from build123d import *

# Parameters (mm, degrees)
SKETCH_1_W                  = 600
SKETCH_1_H                  = 600
EXTRUDE_1_DEPTH             = 780
FILLET_1_R                  = 30
SHELL_1_T                   = 1.2
SKETCH_13_W                 = 348.8
SKETCH_13_H                 = 520
CUT_EXTRUDE_6_DEPTH         = 10
SKETCH_15_W                 = 351.2
SKETCH_15_H                 = 522.4
SKETCH_15_W_2               = 348.8
SKETCH_15_H_2               = 520
EXTRUDE_7_DEPTH             = 15
SKETCH_16_W                 = 351.2
SKETCH_16_H                 = 522.4
SKETCH_16_W_2               = 331.2
SKETCH_16_H_2               = 502.4
EXTRUDE_8_DEPTH             = 1.2
SKETCH_17_W                 = 680
SKETCH_17_H                 = 520
CUT_EXTRUDE_7_DEPTH         = 1.2
SKETCH_19_W                 = 350
SKETCH_19_H                 = 520
CUT_EXTRUDE_8_DEPTH         = 1.2
SKETCH_22_W                 = 352.4
SKETCH_22_H                 = 522.4
SKETCH_22_W_2               = 350
SKETCH_22_H_2               = 520
EXTRUDE_9_DEPTH             = 15
SKETCH_23_W                 = 352.4
SKETCH_23_H                 = 522.4
SKETCH_23_W_2               = 332.4
SKETCH_23_H_2               = 502.4
EXTRUDE_10_DEPTH            = 1.2
SKETCH_24_W                 = 682.4
SKETCH_24_H                 = 522.4
SKETCH_24_W_2               = 680
SKETCH_24_H_2               = 520
EXTRUDE_11_DEPTH            = 15
SKETCH_26_W                 = 682.4
SKETCH_26_H                 = 522.4
SKETCH_26_W_2               = 662.4
SKETCH_26_H_2               = 502.4
EXTRUDE_12_DEPTH            = 1.2
SKETCH_27_W                 = 560
SKETCH_27_H                 = 740
CUT_EXTRUDE_9_DEPTH         = 10
PATTERN_LINEAR_1_COUNT      = 4
PATTERN_LINEAR_1_PITCH      = 166.666666667
HOLE_WIZARD_M6_2_AT_2_COUNT = 2
HOLE_WIZARD_M6_2_AT_2_PITCH = 320
HOLE_WIZARD_M6_2_AT_3_COUNT = 2
HOLE_WIZARD_M6_2_AT_3_PITCH = 640
SKETCH_32_W                 = 678.8
SKETCH_32_H                 = 520
CUT_EXTRUDE_10_DEPTH        = 10
SKETCH_33_W                 = 681.2
SKETCH_33_H                 = 522.4
SKETCH_33_W_2               = 678.8
SKETCH_33_H_2               = 520
EXTRUDE_13_DEPTH            = 15
SKETCH_34_W                 = 681.2
SKETCH_34_H                 = 522.4
SKETCH_34_W_2               = 641.2
SKETCH_34_H_2               = 482.4
EXTRUDE_14_DEPTH            = 1.2
SKETCH_35_R                 = 2.5
EXTRUDE_15_DEPTH            = 20
EXTRUDE_START               = 20
SKETCH_36_R                 = 2.5
EXTRUDE_16_DEPTH            = 20


with BuildPart() as part:
    # 草图1 → 凸台-拉伸1 (new body)
    with BuildSketch(Plane.XY):
        Rectangle(SKETCH_1_W, SKETCH_1_H)
    extrude(amount=EXTRUDE_1_DEPTH)

    # 圆角1
    fillet_1_edges = [part.edges().sort_by_distance(p)[0] for p in [
        (-300, 0, 780),
        (300, 0, 780),
        (-300, 0, 0),
        (300, 0, 0),
    ]]
    fillet(fillet_1_edges, radius=FILLET_1_R)

    # 抽壳1 (no face opened: a closed hollow body)
    add(offset(amount=-SHELL_1_T, mode=Mode.PRIVATE), mode=Mode.SUBTRACT)

    # 草图13 → 切除-拉伸6 (cut)
    with BuildSketch(Plane.XY.offset(780)):
        with Locations((-74.4, 10)):
            Rectangle(SKETCH_13_W, SKETCH_13_H)
    extrude(amount=-CUT_EXTRUDE_6_DEPTH, mode=Mode.SUBTRACT)

    # 草图15 → 凸台-拉伸7 (add)
    with BuildSketch(Plane.XY.offset(780)):
        with Locations((-74.4, 10)):
            Rectangle(SKETCH_15_W, SKETCH_15_H)
        with Locations((-74.4, 10)):
            Rectangle(SKETCH_15_W_2, SKETCH_15_H_2, mode=Mode.SUBTRACT)
    extrude(amount=-EXTRUDE_7_DEPTH)

    # 草图16 → 凸台-拉伸8 (add)
    with BuildSketch(Plane(origin=(0, 0, 765), x_dir=(-1, 0, 0), z_dir=(0, 0, -1))):
        with Locations((74.4, 10)):
            Rectangle(SKETCH_16_W, SKETCH_16_H)
        with Locations((74.4, 10)):
            Rectangle(SKETCH_16_W_2, SKETCH_16_H_2, mode=Mode.SUBTRACT)
    extrude(amount=EXTRUDE_8_DEPTH)

    # 草图17 → 切除-拉伸7 (cut)
    with BuildSketch(Plane(origin=(-300, 0, 0), x_dir=(0, 0, -1), z_dir=(1, 0, 0))):
        with Locations((-390, 10)):
            Rectangle(SKETCH_17_W, SKETCH_17_H)
    extrude(amount=CUT_EXTRUDE_7_DEPTH, mode=Mode.SUBTRACT)

    # 草图19 → 切除-拉伸8 (cut)
    with BuildSketch(Plane(origin=(0, 0, 0), x_dir=(-1, 0, 0), z_dir=(0, 0, -1))):
        with Locations((75, 10)):
            Rectangle(SKETCH_19_W, SKETCH_19_H)
    extrude(amount=-CUT_EXTRUDE_8_DEPTH, mode=Mode.SUBTRACT)

    # 草图22 → 凸台-拉伸9 (add)
    with BuildSketch(Plane(origin=(0, 0, 0), x_dir=(-1, 0, 0), z_dir=(0, 0, -1))):
        with Locations((75, 10)):
            Rectangle(SKETCH_22_W, SKETCH_22_H)
        with Locations((75, 10)):
            Rectangle(SKETCH_22_W_2, SKETCH_22_H_2, mode=Mode.SUBTRACT)
    extrude(amount=-EXTRUDE_9_DEPTH)

    # 草图23 → 凸台-拉伸10 (add)
    with BuildSketch(Plane.XY.offset(15)):
        with Locations((-75, 10)):
            Rectangle(SKETCH_23_W, SKETCH_23_H)
        with Locations((-75, 10)):
            Rectangle(SKETCH_23_W_2, SKETCH_23_H_2, mode=Mode.SUBTRACT)
    extrude(amount=EXTRUDE_10_DEPTH)

    # 草图24 → 凸台-拉伸11 (add)
    with BuildSketch(Plane(origin=(-300, 0, 0), x_dir=(0, 0, -1), z_dir=(1, 0, 0))):
        with Locations((-390, 10)):
            Rectangle(SKETCH_24_W, SKETCH_24_H)
        with Locations((-390, 10)):
            Rectangle(SKETCH_24_W_2, SKETCH_24_H_2, mode=Mode.SUBTRACT)
    extrude(amount=EXTRUDE_11_DEPTH)

    # 草图26 → 凸台-拉伸12 (add)
    with BuildSketch(Plane(origin=(-285, 0, 0), x_dir=(0, 0, -1), z_dir=(1, 0, 0))):
        with Locations((-390, 10)):
            Rectangle(SKETCH_26_W, SKETCH_26_H)
        with Locations((-390, 10)):
            Rectangle(SKETCH_26_W_2, SKETCH_26_H_2, mode=Mode.SUBTRACT)
    extrude(amount=EXTRUDE_12_DEPTH)

    # 草图27 → 切除-拉伸9 (cut)
    with BuildSketch(Plane(origin=(0, 300, 0), x_dir=(1, 0, 0), z_dir=(0, 1, 0))):
        with Locations((0, -390)):
            Rectangle(SKETCH_27_W, SKETCH_27_H)
    extrude(amount=-CUT_EXTRUDE_9_DEPTH, mode=Mode.SUBTRACT)

    # 草图29 → M6 螺纹孔1 (revolve, cut)
    with BuildSketch(Plane(origin=(250, 300, 770), x_dir=(0, 0, 1), z_dir=(1, 0, 0))):
        Polygon((0, 0), (0, 16.502151548), (2.5, 15), (2.5, 0), align=None)
    hole_wizard_m6_1 = revolve(axis=Axis((250, 306.35, 770), (0, -1, 0)), mode=Mode.SUBTRACT)

    # 阵列(线性)1: M6 螺纹孔1 ×4
    with Locations(*[(-i * PATTERN_LINEAR_1_PITCH, 0, 0) for i in range(1, PATTERN_LINEAR_1_COUNT)]):
        add(hole_wizard_m6_1, mode=Mode.SUBTRACT)

    # 镜向1: M6 螺纹孔1 across plane
    add(hole_wizard_m6_1.mirror(Plane(origin=(0, 0, 390), x_dir=(1, 0, 0), z_dir=(0, 0, -1))), mode=Mode.SUBTRACT)

    # 镜向1 copy 1 sketch → 镜向1 copy 1 (revolve, cut)
    with BuildSketch(Plane(origin=(83.333333333, 300, 10), x_dir=(0, 0, -1), z_dir=(1, 0, 0))):
        Polygon((0, 0), (0, -16.502151548), (2.5, -15), (2.5, 0), align=None)
    revolve(axis=Axis((83.333333333, 306.35, 10), (0, 1, 0)), mode=Mode.SUBTRACT)

    # 镜向1 copy 2 sketch → 镜向1 copy 2 (revolve, cut)
    with BuildSketch(Plane(origin=(-83.333333333, 300, 10), x_dir=(0, 0, -1), z_dir=(1, 0, 0))):
        Polygon((0, 0), (0, -16.502151548), (2.5, -15), (2.5, 0), align=None)
    revolve(axis=Axis((-83.333333333, 306.35, 10), (0, 1, 0)), mode=Mode.SUBTRACT)

    # 镜向1 copy 3 sketch → 镜向1 copy 3 (revolve, cut)
    with BuildSketch(Plane(origin=(-250, 300, 10), x_dir=(0, 0, -1), z_dir=(1, 0, 0))):
        Polygon((0, 0), (0, -16.502151548), (2.5, -15), (2.5, 0), align=None)
    revolve(axis=Axis((-250, 306.35, 10), (0, 1, 0)), mode=Mode.SUBTRACT)

    # 草图31 → M6 螺纹孔2 (revolve, cut)
    with BuildSketch(Plane(origin=(290, 300, 710), x_dir=(0, 0, 1), z_dir=(1, 0, 0))):
        Polygon((0, 0), (0, 16.502151548), (2.5, 15), (2.5, 0), align=None)
    hole_wizard_m6_2 = revolve(axis=Axis((290, 306.35, 710), (0, -1, 0)), mode=Mode.SUBTRACT)

    # M6 螺纹孔2 at 2: M6 螺纹孔2 ×2
    with Locations(*[(0, 0, -i * HOLE_WIZARD_M6_2_AT_2_PITCH) for i in range(1, HOLE_WIZARD_M6_2_AT_2_COUNT)]):
        add(hole_wizard_m6_2, mode=Mode.SUBTRACT)

    # M6 螺纹孔2 at 3: M6 螺纹孔2 ×2
    with Locations(*[(0, 0, -i * HOLE_WIZARD_M6_2_AT_3_PITCH) for i in range(1, HOLE_WIZARD_M6_2_AT_3_COUNT)]):
        add(hole_wizard_m6_2, mode=Mode.SUBTRACT)

    # 镜向2: M6 螺纹孔2 across plane
    add(hole_wizard_m6_2.mirror(Plane(origin=(0, 0, 0), x_dir=(0, 0, 1), z_dir=(1, 0, 0))), mode=Mode.SUBTRACT)

    # 镜向2 copy 1 sketch → 镜向2 copy 1 (revolve, cut)
    with BuildSketch(Plane(origin=(-290, 300, 390), x_dir=(0, 0, 1), z_dir=(-1, 0, 0))):
        Polygon((0, 0), (0, -16.502151548), (2.5, -15), (2.5, 0), align=None)
    revolve(axis=Axis((-290, 306.35, 390), (0, 1, 0)), mode=Mode.SUBTRACT)

    # 镜向2 copy 2 sketch → 镜向2 copy 2 (revolve, cut)
    with BuildSketch(Plane(origin=(-290, 300, 70), x_dir=(0, 0, 1), z_dir=(-1, 0, 0))):
        Polygon((0, 0), (0, -16.502151548), (2.5, -15), (2.5, 0), align=None)
    revolve(axis=Axis((-290, 306.35, 70), (0, 1, 0)), mode=Mode.SUBTRACT)

    # 镜向3: M6 螺纹孔2 across plane
    add(hole_wizard_m6_2.mirror(Plane(origin=(0, 0, 0), x_dir=(0, 0, 1), z_dir=(1, 0, 0))), mode=Mode.SUBTRACT)

    # 镜向3 copy 1 sketch → 镜向3 copy 1 (revolve, cut)
    with BuildSketch(Plane(origin=(-290, 300, 390), x_dir=(0, 0, 1), z_dir=(-1, 0, 0))):
        Polygon((0, 0), (0, -16.502151548), (2.5, -15), (2.5, 0), align=None)
    revolve(axis=Axis((-290, 306.35, 390), (0, 1, 0)), mode=Mode.SUBTRACT)

    # 镜向3 copy 2 sketch → 镜向3 copy 2 (revolve, cut)
    with BuildSketch(Plane(origin=(-290, 300, 70), x_dir=(0, 0, 1), z_dir=(-1, 0, 0))):
        Polygon((0, 0), (0, -16.502151548), (2.5, -15), (2.5, 0), align=None)
    revolve(axis=Axis((-290, 306.35, 70), (0, 1, 0)), mode=Mode.SUBTRACT)

    # 草图32 → 切除-拉伸10 (cut)
    with BuildSketch(Plane(origin=(300, 0, 0), x_dir=(0, 0, -1), z_dir=(1, 0, 0))):
        with Locations((-390.6, 10)):
            Rectangle(SKETCH_32_W, SKETCH_32_H)
    extrude(amount=-CUT_EXTRUDE_10_DEPTH, mode=Mode.SUBTRACT)

    # 草图33 → 凸台-拉伸13 (add)
    with BuildSketch(Plane(origin=(300, 0, 0), x_dir=(0, 0, -1), z_dir=(1, 0, 0))):
        with Locations((-390.6, 10)):
            Rectangle(SKETCH_33_W, SKETCH_33_H)
        with Locations((-390.6, 10)):
            Rectangle(SKETCH_33_W_2, SKETCH_33_H_2, mode=Mode.SUBTRACT)
    extrude(amount=-EXTRUDE_13_DEPTH)

    # 草图34 → 凸台-拉伸14 (add)
    with BuildSketch(Plane.ZY.offset(-285)):
        with Locations((390.6, 10)):
            Rectangle(SKETCH_34_W, SKETCH_34_H)
        with Locations((390.6, 10)):
            Rectangle(SKETCH_34_W_2, SKETCH_34_H_2, mode=Mode.SUBTRACT)
    extrude(amount=EXTRUDE_14_DEPTH)

    # 草图35 → 凸台-拉伸15 (add)
    with BuildSketch(Plane(origin=(0, 0, 778.8), x_dir=(-1, 0, 0), z_dir=(0, 0, -1))):
        with Locations((-120, 120)):
            Circle(SKETCH_35_R)
        with Locations((-120, -230)):
            Circle(SKETCH_35_R)
    extrude(amount=EXTRUDE_15_DEPTH)

    # 草图36 → 凸台-拉伸16 (add)
    with BuildSketch(Plane.XY.offset(1.2).offset(EXTRUDE_START)):
        with Locations(Location((120, 120, 0), (0, 0, 180))):
            Circle(SKETCH_36_R)
        with Locations(Location((120, -230, 0), (0, 0, 180))):
            Circle(SKETCH_36_R)
    extrude(amount=-EXTRUDE_16_DEPTH)


solid = part.part
Could you check a few things on this model? Use its own coordinates, in mm. A direction names the side the tool comes from. Coordinates: 2 decimals unless noted, no trailing zeros. Order: outer loops, then holes, each group sorted by start corner. A loop starts at its lowest first (then second) coordinate and runs counter-clockwise, first axis right, second up. Notation, with made-up numbers: (74, 17) - (97, 17) arc R15 ccw to (97, 23) - close; hole circle Ø10 at (44.5, 44.5). An arc over 180 degrees is marked (long way). Answer in a Markdown table with one row per item. Add a question column.
(1) On a 3-axis mill with a long thin cutter (end or side, diameter ignored), from which of +Z, -Z, +X, -X, +Y, -Y can I reach the whole of each face in a straight line? I mean faces 1 (the face through (-285, 262, 392)), 2 (the face through (291.445, 4.2, 770.979)), 3 (the face through (298.8, -267, 388)), 4 (the face through (94, 88, 765)), 5 (the face through (-300, -268, 388)). Say none if no direction works.
(2) I need wall thicknesses on L1, parallel to Z at x = 290, y = 299.75; L2, parallel to Z at x = 250, y = 299; L3, parallel to X at y = 299.4, z = 10. Which ranges of each line are inside material? Lowest first, please.
(3) If we mould it in two halves opening along Z, with no side actions, what happens to faces 6 (the face through (300, -268, 388)), 7 (the face through (-244, 88, 15)), 8 (the face through (116, 4, 780)), 9 (the face through (-245, 89, 16.2))? For each: released by +Z, released by -Z, zero draft, split by the parting line, or undercut.
(4) If we section it at B-B, the plane z = 529: State how many separate pieces and enclosed holes the cut face has, then the cut area to 3 significant figures.
(5) Will these pins go through, and if not, where does the flat tip stop? pin 1 (4.5 mm diameter, centred on x = -294.5, y = -99.5, fed in from +Z); pin 2 (10 mm diameter, centred on x = 30.5, z = 344.5, fed in from +Y); pin 3 (16.5 mm diameter, centred on y = -30.5, z = 774.5, fed in from +X).
(6) If we section it at A-A, the plane x = 153: Please give me the cut outline in (y, z).
Results are:
| question | item | result |
|---|---|---|
| 1 | face 1 | -X |
| 1 | face 2 | +Z, +X, +Y, -Y |
| 1 | face 3 | none |
| 1 | face 4 | +Z |
| 1 | face 5 | +Z, -Z, -X, +Y, -Y |
| 2 | L1 | z = 7.64 to 67.5, 72.5 to 387.5, 392.5 to 707.5, 712.5 to 772.36 |
| 2 | L2 | z = 0 to 7.5, 12.5 to 20, 760 to 767.5, 772.5 to 780 |
| 2 | L3 | x = -292.36 to -252.5, -247.5 to -85.83, -80.83 to 80.83, 85.83 to 247.5, 252.5 to 292.36 |
| 3 | face 6 | zero draft |
| 3 | face 7 | released by -Z |
| 3 | face 8 | released by +Z |
| 3 | face 9 | undercut |
| 4 | separate pieces | 3 |
| 4 | enclosed holes | 0 |
| 4 | area | 1,090 mm2 |
| 5 | pin 1 | stops at z = 770.12 |
| 5 | pin 2 | stops at y = -298.8 |
| 5 | pin 3 | stops at x = 295.22 |
| 6 | outline | (-300, 0) - (300, 0) - (300, 20) - (298.8, 20) - (298.8, 1.2) - (-298.8, 1.2) - (-298.8, 778.8) - (298.8, 778.8) - (298.8, 760) - (300, 760) - (300, 780) - (-300, 780) - close |
